Build history of the part. All positions in model axes, mm. Face numbers are marked on the shaded views. A direction names the side the tool comes from. Give positions to 0.01 mm unless a question says otherwise; leave off trailing zeros. Order: outer loops, then holes, each group sorted by start corner. A loop starts at its lowest first (then second) coordinate and runs counter-clockwise, first axis right, second up. Notation, with made-up numbers: (85, 3) -> (135, 3) arc R9 cw to (135, 8) -> close; hole circle Ø9 at (64, -28). An arc over 180 degrees is marked (long way). One line per question, with ' | ' between items. Start each with the question number.
(1) Drill centre lines: L1, parallel to X at y = 71, z = 229; L2, parallel to Y at x = 183, z = 32.5; L3, parallel to Z at x = 453.5, y = 202.5. Where is each one in solid material? Low to high. Write a range as from..to.
(2) Cut at A-A (z = 205). Give the cut face in (x, y).
(3) Pull direction X, two halves, no side cores. Call the marked faces 1, 2, 3 and 4: +X half, -X half, draft (parallel to the pull), parting line (faces both ways), or undercut.
(4) Pin check, flat tip, straight feed: pin 1 Ø3 at (x, y) = (262.5, 251) entering from +Z. Stop position of the tip, or through.
(5) Cut at C-C (y = 303). Give the cut face in (x, z), then the cut area to 3 significant figures.
(6) Which spindle directions (+Z, -Z, +X, -X, +Y, -Y) get a long thin tool onto all of the face, cutting with end or side? Do the marked faces 5 and 6. Say none if no direction does.
(7) Cut at B-B (x = 646.5). Give the cut face in (y, z).
from build123d import *

# Parameters (mm, degrees)
F0_W     = 800
F0_H     = 400
F0_W_2   = 750
F0_H_2   = 350
F1_DEPTH = 300
F2_R     = 15
F4_DEPTH = 25


with BuildPart() as f1:
    # F0 (on Top) → F1 (new body)
    with BuildSketch(Plane.XY):
        with Locations((400, 200)):
            Rectangle(F0_W, F0_H)
        with Locations((400, 200)):
            Rectangle(F0_W_2, F0_H_2, mode=Mode.SUBTRACT)
    extrude(amount=F1_DEPTH)

    # F2
    f2_edges = [f1.edges().sort_by_distance(p)[0] for p in [
        (0, 0, 150),
        (800, 0, 150),
        (0, 400, 150),
        (800, 400, 150),
        (25, 25, 150),
        (25, 375, 150),
        (775, 25, 150),
        (775, 375, 150),
    ]]
    fillet(f2_edges, radius=F2_R)

    # F3 (on face) → F4 (join)
    with BuildSketch(Plane(origin=(0, 0, 0), x_dir=(1, 0, 0), z_dir=(0, 0, -1))):
        with BuildLine():
            ThreePointArc((800, -15), (795.606602, -4.393398), (785, 0))
            Line((785, 0), (15, 0))
            ThreePointArc((15, 0), (4.393398, -4.393398), (0, -15))
            Line((0, -15), (0, -385))
            ThreePointArc((0, -385), (4.393398, -395.606602), (15, -400))
            Line((15, -400), (785, -400))
            ThreePointArc((785, -400), (795.606602, -395.606602), (800, -385))
            Line((800, -385), (800, -15))
        make_face()
    extrude(amount=F4_DEPTH)


solid = f1.part
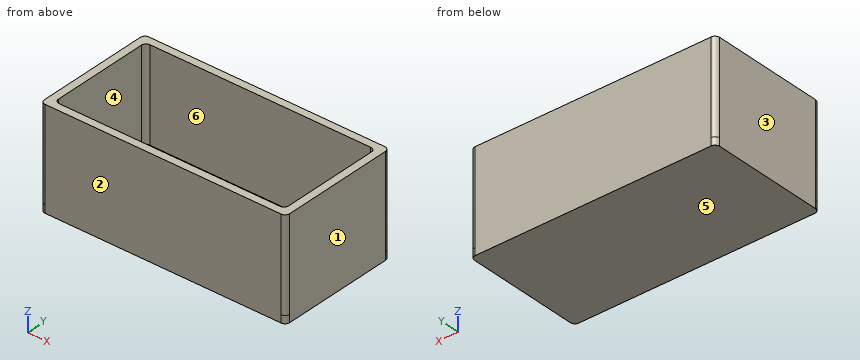
Result set:
1) L1: x = 0..25, 775..800 | L2: y = 0..25, 375..400 | L3: z = -25..0
2) outline: (0, 15) arc R15 ccw to (15, 0) -> (785, 0) arc R15 ccw to (800, 15) -> (800, 385) arc R15 ccw to (785, 400) -> (15, 400) arc R15 ccw to (0, 385) -> close; hole (25, 40) arc R15 ccw to (40, 25) -> (760, 25) arc R15 ccw to (775, 40) -> (775, 360) arc R15 ccw to (760, 375) -> (40, 375) arc R15 ccw to (25, 360) -> close
3) face 1: +X half | face 2: draft | face 3: -X half | face 4: undercut
4) pin 1: stops at z = 0
5) outline: (0, -25) -> (800, -25) -> (800, 300) -> (775, 300) -> (775, 0) -> (25, 0) -> (25, 300) -> (0, 300) -> close | area: 35,000 mm2
6) face 5: -Z, +X, -X, +Y, -Y | face 6: +Z
7) outline: (0, -25) -> (400, -25) -> (400, 300) -> (375, 300) -> (375, 0) -> (25, 0) -> (25, 300) -> (0, 300) -> close
